The listing builds one solid part. Answer for the finished solid, in the listing's coordinates (mm). A direction names the side the tool comes from. Coordinates: 2 decimals unless noted, no trailing zeros. Order: outer loops, then holes, each group sorted by start corner. A loop starts at its lowest first (then second) coordinate and runs counter-clockwise, first axis right, second up. Notation, with made-up numbers: (70, 25.25) -> (118, 25.25) arc R15 cw to (118, 31.25) -> close; hole circle Ø10 at (1.5, 74). An arc over 180 degrees is marked (long way). Answer in a Markdown table with one row per item.
```python
from build123d import *

# Parameters (mm, degrees)
CYLINDER015_R          = 2
CYLINDER015_DEPTH      = 15
CYLINDER015_ROLL_ANGLE = 90
CYLINDER007_R          = 2
CYLINDER007_DEPTH      = 15
CYLINDER006_R          = 2
CYLINDER006_DEPTH      = 15
CYLINDER005_R          = 2
CYLINDER005_DEPTH      = 15
CYLINDER004_R          = 2
CYLINDER004_DEPTH      = 15
CYLINDER003_R          = 2
CYLINDER003_DEPTH      = 15
CYLINDER003_ROLL_ANGLE = 90
CYLINDER002_R          = 2
CYLINDER002_DEPTH      = 15
CYLINDER002_ROLL_ANGLE = 90
CYLINDER001_R          = 2
CYLINDER001_DEPTH      = 15
CYLINDER001_ROLL_ANGLE = 90
CYLINDER_R             = 2
CYLINDER_DEPTH         = 15
CYLINDER_ROLL_ANGLE    = 90
PAD002_DEPTH           = 40.3
BOX_W                  = 40.3
BOX_H                  = 15
BOX_DEPTH              = 25
PAD003_DEPTH           = 55.26
FILLET_R               = 3
FILLET001_R            = 1.5
FILLET002_R            = 2
FILLET005_R            = 5


with BuildPart() as cilindro015:
    # Cylinder015 → Cylinder015 (new body)
    with BuildSketch(Plane.XY):
        Circle(CYLINDER015_R)
    extrude(amount=CYLINDER015_DEPTH)


with BuildPart() as cilindro015_1:
    # Cylinder015 roll: moved
    add(cilindro015.part.rotate(Axis((0, 0, 0), (1, 0, 0)), CYLINDER015_ROLL_ANGLE))


with BuildPart() as cilindro015_2:
    # Cylinder015 placement: moved
    add(cilindro015_1.part.moved(Location((-24.48, 4.65, 15.01))))


with BuildPart() as cilindro007:
    # Cylinder007 → Cylinder007 (new body)
    with BuildSketch(Plane(origin=(24.48, 10.01, -12.65), x_dir=(1, 0, 0), z_dir=(0, 0, 1))):
        Circle(CYLINDER007_R)
    extrude(amount=CYLINDER007_DEPTH)


with BuildPart() as cilindro006:
    # Cylinder006 → Cylinder006 (new body)
    with BuildSketch(Plane(origin=(-24.48, -0.01, -12.65), x_dir=(1, 0, 0), z_dir=(0, 0, 1))):
        Circle(CYLINDER006_R)
    extrude(amount=CYLINDER006_DEPTH)


with BuildPart() as cilindro005:
    # Cylinder005 → Cylinder005 (new body)
    with BuildSketch(Plane(origin=(24.48, -0.01, -12.65), x_dir=(1, 0, 0), z_dir=(0, 0, 1))):
        Circle(CYLINDER005_R)
    extrude(amount=CYLINDER005_DEPTH)


with BuildPart() as cilindro004:
    # Cylinder004 → Cylinder004 (new body)
    with BuildSketch(Plane(origin=(-24.48, 10.01, -12.65), x_dir=(1, 0, 0), z_dir=(0, 0, 1))):
        Circle(CYLINDER004_R)
    extrude(amount=CYLINDER004_DEPTH)


with BuildPart() as cilindro003:
    # Cylinder003 → Cylinder003 (new body)
    with BuildSketch(Plane.XY):
        Circle(CYLINDER003_R)
    extrude(amount=CYLINDER003_DEPTH)


with BuildPart() as cilindro003_1:
    # Cylinder003 roll: moved
    add(cilindro003.part.rotate(Axis((0, 0, 0), (1, 0, 0)), CYLINDER003_ROLL_ANGLE))


with BuildPart() as cilindro003_2:
    # Cylinder003 placement: moved
    add(cilindro003_1.part.moved(Location((-24.48, 4.65, 4.99))))


with BuildPart() as cilindro002:
    # Cylinder002 → Cylinder002 (new body)
    with BuildSketch(Plane.XY):
        Circle(CYLINDER002_R)
    extrude(amount=CYLINDER002_DEPTH)


with BuildPart() as cilindro002_1:
    # Cylinder002 roll: moved
    add(cilindro002.part.rotate(Axis((0, 0, 0), (1, 0, 0)), CYLINDER002_ROLL_ANGLE))


with BuildPart() as cilindro002_2:
    # Cylinder002 placement: moved
    add(cilindro002_1.part.moved(Location((-24.48, 4.65, 15.01))))


with BuildPart() as cilindro001:
    # Cylinder001 → Cylinder001 (new body)
    with BuildSketch(Plane.XY):
        Circle(CYLINDER001_R)
    extrude(amount=CYLINDER001_DEPTH)


with BuildPart() as cilindro001_1:
    # Cylinder001 roll: moved
    add(cilindro001.part.rotate(Axis((0, 0, 0), (1, 0, 0)), CYLINDER001_ROLL_ANGLE))


with BuildPart() as cilindro001_2:
    # Cylinder001 placement: moved
    add(cilindro001_1.part.moved(Location((24.48, 4.65, 4.99))))


with BuildPart() as cilindro:
    # Cylinder → Cylinder (new body)
    with BuildSketch(Plane.XY):
        Circle(CYLINDER_R)
    extrude(amount=CYLINDER_DEPTH)


with BuildPart() as cilindro_1:
    # Cylinder roll: moved
    add(cilindro.part.rotate(Axis((0, 0, 0), (1, 0, 0)), CYLINDER_ROLL_ANGLE))


with BuildPart() as cilindro_2:
    # Cylinder placement: moved
    add(cilindro_1.part.moved(Location((24.48, 4.65, 15.01))))


with BuildPart() as pad002:
    # Sketch002 → Pad002 (new body)
    with BuildSketch(Plane.YZ.offset(-20.15)):
        Polygon((17.3, 18.5), (21.3, 18.5), (21.3, -4.5), (-7.7, -4.5), (-7.7, -0.5), (17.3, -0.5), align=None)
    extrude(amount=PAD002_DEPTH)


with BuildPart() as cubo:
    # Box → Box (new body)
    with BuildSketch(Plane(origin=(-20.15, -12.7, -2.5), x_dir=(1, 0, 0), z_dir=(0, 0, 1))):
        with Locations((20.15, 7.5)):
            Rectangle(BOX_W, BOX_H)
    extrude(amount=BOX_DEPTH)


with BuildPart() as pieza1v1:
    # Sketch003 → Pad003 (new body)
    with BuildSketch(Plane.YZ.offset(-27.63)):
        Polygon((-7.7, -4.5), (16.3, -4.5), (16.3, -0.5), (-3.7, -0.5), (-3.7, 18.2), (-7.7, 18.2), align=None)
    extrude(amount=PAD003_DEPTH)

    # Cut: cut Cubo
    add(cubo.part, mode=Mode.SUBTRACT)

    # Fusion: union Pad002
    add(pad002.part)

    # Fillet
    fillet_edges = [pieza1v1.edges().sort_by_distance(p)[0] for p in [
        (-23.89, -3.7, -0.5),
        (23.89, -3.7, -0.5),
    ]]
    fillet(fillet_edges, radius=FILLET_R)

    # Fillet001
    fillet001_edges = [pieza1v1.edges().sort_by_distance(p)[0] for p in [
        (0, -7.7, -4.5),
    ]]
    fillet(fillet001_edges, radius=FILLET001_R)

    # Fillet002
    fillet002_edges = [pieza1v1.edges().sort_by_distance(p)[0] for p in [
        (0, 17.3, -0.5),
    ]]
    fillet(fillet002_edges, radius=FILLET002_R)

    # Fillet005
    fillet005_edges = [pieza1v1.edges().sort_by_distance(p)[0] for p in [
        (0, 21.3, -4.5),
    ]]
    fillet(fillet005_edges, radius=FILLET005_R)

    # Cut015: cut Cilindro
    add(cilindro_2.part, mode=Mode.SUBTRACT)

    # Cut016: cut Cilindro001
    add(cilindro001_2.part, mode=Mode.SUBTRACT)

    # Cut017: cut Cilindro002
    add(cilindro002_2.part, mode=Mode.SUBTRACT)

    # Cut018: cut Cilindro003
    add(cilindro003_2.part, mode=Mode.SUBTRACT)

    # Cut019: cut Cilindro004
    add(cilindro004.part, mode=Mode.SUBTRACT)

    # Cut020: cut Cilindro005
    add(cilindro005.part, mode=Mode.SUBTRACT)

    # Cut021: cut Cilindro006
    add(cilindro006.part, mode=Mode.SUBTRACT)

    # Cut022: cut Cilindro007
    add(cilindro007.part, mode=Mode.SUBTRACT)

    # Cut023: cut Cilindro015
    add(cilindro015_2.part, mode=Mode.SUBTRACT)


with BuildPart() as pieza1v1_1:
    # Cut023 placement: moved
    add(pieza1v1.part.moved(Location((10.1, -0.05, -10))))


solid = pieza1v1_1.part
```
(1) Flat-ended cylindrical pins translate along their axes: pin 1 (1.3 mm diameter, centred on x = 35, z = -11.5, fed in from +Y); pin 2 (8 mm diameter, centred on x = 25, y = 10.5, fed in from +Z); pin 3 (1.5 mm diameter, centred on y = 18, z = 2.5, fed in from -X); pin 4 (8 mm diameter, centred on y = 4, z = -3.5, fed in from -X). Find the tip coordinate at first contact, or state that the pin passes through.
Check values:
| item | result |
|---|---|
| pin 1 | y = 16.25 |
| pin 2 | z = -10.5 |
| pin 3 | x = -10.05 |
| pin 4 | through |
(2) A cutting plane is placed at D-D, the plane y = 10.5. Determine the outline of the cut face in (x, z), then the cut area to 3 significant figures.
Check values:
| item | result |
|---|---|
| outline | (-17.53, -14.5) -> (-16.31, -14.5) -> (-16.31, -10.5) -> (-17.53, -10.5) -> close; (-12.45, -14.5) -> (32.65, -14.5) -> (32.65, -10.5) -> (-12.45, -10.5) -> close; (36.51, -14.5) -> (37.73, -14.5) -> (37.73, -10.5) -> (36.51, -10.5) -> close |
| area | 190 mm² |
(3) Find the intervals of material crossed by line 1 along Y through (x, z) = (-14.38, -12.45); line 2 along Z through (x, y) = (34.58, -4.95); line 3 along Y through (x, z) = (1.5, 4.5), in increasing order. Write a range as from..to.
Check values:
| item | result |
|---|---|
| line 1 | -7.75..-2.06, 1.94..7.96, 11.96..16.25 |
| line 2 | -14.5..-7.01, -3.01..3.01, 7.01..8.2 |
| line 3 | 17.25..21.25 |
(4) For a pull along Z with two mould halves and no side action, classify faces 1 (the cylindrical face through (-14.814, -2.012, -12.38)), 2 (the cylindrical face through (10.49, 16.65, -9.93)), 3 (the cylindrical face through (32.582, -5.722, 5.098)) as released by +Z, released by -Z, zero draft, split by the parting line, or undercut.
Check values:
| item | result |
|---|---|
| face 1 | zero draft |
| face 2 | released by +Z |
| face 3 | undercut |
(5) A cutting plane is placed at A-A, the plane z = 5.01. Determine the outline of the cut face in (x, y).
Check values:
| item | result |
|---|---|
| outline | (-17.53, -7.75) -> (-16.38, -7.75) -> (-16.38, -3.75) -> (-17.53, -3.75) -> close; (-12.38, -7.75) -> (-10.05, -7.75) -> (-10.05, -3.75) -> (-12.38, -3.75) -> close; (-10.05, 17.25) -> (30.25, 17.25) -> (30.25, 21.25) -> (-10.05, 21.25) -> close; (30.25, -7.75) -> (32.58, -7.75) -> (32.58, -3.75) -> (30.25, -3.75) -> close; (36.58, -7.75) -> (37.73, -7.75) -> (37.73, -3.75) -> (36.58, -3.75) -> close |
(6) A cutting plane is placed at C-C, the plane x = 2. Determine the outline of the cut face in (y, z).
Check values:
| item | result |
|---|---|
| outline | (-7.75, -13) arc R1.5 ccw to (-6.25, -14.5) -> (16.25, -14.5) arc R5 ccw to (21.25, -9.5) -> (21.25, 8.5) -> (17.25, 8.5) -> (17.25, -8.5) arc R2 cw to (15.25, -10.5) -> (-7.75, -10.5) -> close |
(7) A cutting plane is placed at B-B, the plane x = 34.58. Determine the outline of the cut face in (y, z), then the cut area to 3 significant figures.
Check values:
| item | result |
|---|---|
| outline | (-7.75, -13) arc R1.5 ccw to (-6.25, -14.5) -> (-2.06, -14.5) -> (-2.06, -10.2) arc R3 cw to (-3.75, -7.5) -> (-3.75, -7.01) -> (-7.75, -7.01) -> close; (-7.75, -3.01) -> (-3.75, -3.01) -> (-3.75, 3.01) -> (-7.75, 3.01) -> close; (-7.75, 7.01) -> (-3.75, 7.01) -> (-3.75, 8.2) -> (-7.75, 8.2) -> close; (1.94, -14.5) -> (7.96, -14.5) -> (7.96, -10.5) -> (1.94, -10.5) -> close; (11.96, -14.5) -> (16.25, -14.5) -> (16.25, -10.23) arc R2 cw to (15.25, -10.5) -> (11.96, -10.5) -> close |
| area | 108 mm² |
(8) Which of the six approach directions +Z, -Z, +X, -X, +Y, -Y give full straight-line access (tool end or side, diameter ignored) to faces 4 (the flat face through (30.25, 19, -3)), 5 (the cylindrical face through (34.04, -2.89, -9.6)), 6 (the flat face through (34, -3.75, 0))?
Check values:
| item | result |
|---|---|
| face 4 | +Z, -Z, +X, +Y |
| face 5 | +Z, +X, -X |
| face 6 | +Z, +X, -X, +Y |
